Verification items for the finished model (mm, model axes). A direction names the side the tool comes from. Round coordinates to 2 decimals unless told otherwise and drop trailing zeros. Write each loop counter-clockwise with the first axis right and the second up, starting at its lowest first coordinate (ties: lowest second). Pieces come first, ordered by that corner, then holes. Notation, with made-up numbers: M 19,41.5 L 35,41.5 A20 cw 35,57.5 Z; hole C 79.25,-15 d5. An arc over 180 degrees is marked long. Answer in a Markdown table with one row per item. Add a question column.
1. Sectioned sample at A-A on x = 55. Record the cut outline in (y, z), plus the area to 3 significant figures.
2. Material ranges on probe 1 along Y at (x, z) = (105, 3.5); probe 2 along Y at (x, z) = (55, 2.5); probe 3 along Z at (x, y) = (40, 15.5), recorded low to high.
3. Sectioned sample at D-D on x = 70. Record the cut outline in (y, z).
4. Go/stop test with flat-tipped pins: pin 1 Ø5 at (x, z) = (70.5, 7) entering from +Y; pin 2 Ø12 at (x, y) = (53.5, 13.5) entering from +Z; pin 3 Ø3.5 at (x, y) = (105, 10) entering from -Z. Record where each tip stops, or that it passes through.
5. Sectioned sample at C-C on z = 2. Record the cut outline in (x, y), plus the area to 3 significant figures.
6. Draft check along Z on faces 1 (the flat face through (47.35, 12, 7)), 2 (the cylindrical face through (72.4, 17.6, 4.2)), 3 (the flat face through (54, 13, 0)), 4 (the cylindrical face through (43, 18, 6)). Enter one of: pulls with the +Z half, pulls with the -Z half, needs draft (parallel to the pull), parting line crosses it, or undercut.
7. Sectioned sample at B-B on y = 5.5. Record the cut outline in (x, z), plus the area to 3 significant figures.
8. Set-up check for faces 5 (the flat face through (40, 10, 6)), 6 (the flat face through (54.2, 0, 3.8)), 7 (the flat face through (62.65, 12, 7)): record each of +Z, -Z, +X, -X, +Y, -Y from which the full face is reachable in a straight line by a thin tool's end or side.
```python
from build123d import *

# Parameters (mm, degrees)
ESQUISSE1_W             = 110
ESQUISSE1_H             = 25
ESQUISSE1_R             = 2
BOSS_EXTRU_1_DEPTH      = 10
ESQUISSE2_W             = 15.3
ESQUISSE2_H             = 25
ENL_V_MAT_EXTRU_1_DEPTH = 6
ESQUISSE3_R             = 3
ENL_V_MAT_EXTRU_2_DEPTH = 15


with BuildPart() as part:
    # Esquisse1 → Boss.-Extru.1 (new body)
    with BuildSketch(Plane.XY):
        with Locations((55, 12.5)):
            Rectangle(ESQUISSE1_W, ESQUISSE1_H)
        with Locations((5, 20)):
            Circle(ESQUISSE1_R, mode=Mode.SUBTRACT)
        with Locations((5, 10)):
            Circle(ESQUISSE1_R, mode=Mode.SUBTRACT)
        with Locations((105, 20)):
            Circle(ESQUISSE1_R, mode=Mode.SUBTRACT)
        with Locations((105, 10)):
            Circle(ESQUISSE1_R, mode=Mode.SUBTRACT)
        with Locations((55, 19.5)):
            Circle(ESQUISSE1_R, mode=Mode.SUBTRACT)
        with Locations((55, 5.5)):
            Circle(ESQUISSE1_R, mode=Mode.SUBTRACT)
    extrude(amount=BOSS_EXTRU_1_DEPTH)

    # Esquisse2 → Enlèv. mat.-Extru.1 (cut)
    with BuildSketch(Plane.XY.offset(10)):
        with Locations((55, 12.5)):
            Rectangle(ESQUISSE2_W, ESQUISSE2_H)
    extrude(amount=-ENL_V_MAT_EXTRU_1_DEPTH, mode=Mode.SUBTRACT)

    # Esquisse3 → Enlèv. mat.-Extru.2 (cut)
    with BuildSketch(Plane(origin=(0, 25, 0), x_dir=(1, 0, 0), z_dir=(0, 1, 0))):
        with Locations(Location((70, -6, 0), (0, 0, 180))):
            Circle(ESQUISSE3_R)
        with Locations(Location((40, -6, 0), (0, 0, 180))):
            Circle(ESQUISSE3_R)
    extrude(amount=-ENL_V_MAT_EXTRU_2_DEPTH, mode=Mode.SUBTRACT)


solid = part.part
```
Geometry check:
| question | item | result |
|---|---|---|
| 1 | outline | M 0,0 L 3.5,0 L 3.5,4 L 0,4 Z; M 7.5,0 L 17.5,0 L 17.5,4 L 7.5,4 Z; M 21.5,0 L 25,0 L 25,4 L 21.5,4 Z |
| 1 | area | 68.0 mm2 |
| 2 | probe 1 | y = 0 to 8, 12 to 18, 22 to 25 |
| 2 | probe 2 | y = 0 to 3.5, 7.5 to 17.5, 21.5 to 25 |
| 2 | probe 3 | z = 0 to 3, 9 to 10 |
| 3 | outline | M 0,0 L 25,0 L 25,3 L 10,3 L 10,9 L 25,9 L 25,10 L 0,10 Z |
| 4 | pin 1 | stops at y = 25 |
| 4 | pin 2 | stops at z = 4 |
| 4 | pin 3 | passes through |
| 5 | outline | M 0,0 L 110,0 L 110,25 L 0,25 Z; hole C 5,10 d4; hole C 5,20 d4; hole C 55,5.5 d4; hole C 55,19.5 d4; hole C 105,10 d4; hole C 105,20 d4 |
| 5 | area | 2,670 mm2 |
| 6 | face 1 | needs draft |
| 6 | face 2 | undercut |
| 6 | face 3 | pulls with the -Z half |
| 6 | face 4 | undercut |
| 7 | outline | M 0,0 L 53,0 L 53,4 L 47.35,4 L 47.35,10 L 0,10 Z; M 57,0 L 110,0 L 110,10 L 62.65,10 L 62.65,4 L 57,4 Z |
| 7 | area | 992 mm2 |
| 8 | face 5 | +Y |
| 8 | face 6 | +Z, -Z, +X, -X, -Y |
| 8 | face 7 | +Z, +Y, -Y |
